Part model, mm, in its own coordinate system. A direction names the side the tool comes from. Round coordinates to 2 decimals unless told otherwise and drop trailing zeros. Order: outer loops, then holes, each group sorted by start corner. A loop starts at its lowest first (then second) coordinate and runs counter-clockwise, first axis right, second up. Notation, with made-up numbers: (-2.5, 41.25) - (41.5, 41.25) arc R18 ccw to (41.5, 67.25) - close; hole circle Ø8 at (26, 66). An arc over 180 degrees is marked (long way). Answer as a JSON object with one key per item and string values.
```python
from build123d import *

# Parameters (mm, degrees)
SKETCH1_R           = 200
SKETCH1_R_2         = 195
BOSS_EXTRUDE1_DEPTH = 137
SKETCH2_W           = 16
SKETCH2_H           = 10
CUT_EXTRUDE1_DEPTH  = 70.5


with BuildPart() as part:
    # Sketch1 → Boss-Extrude1 (new body)
    with BuildSketch(Plane(origin=(0, 0, 0), x_dir=(1, 0, 0), z_dir=(0, 1, 0))):
        with Locations(Location((0, 0, 0), (0, 0, 270))):
            Circle(SKETCH1_R)
        with Locations(Location((0, 0, 0), (0, 0, 270))):
            Circle(SKETCH1_R_2, mode=Mode.SUBTRACT)
    extrude(amount=BOSS_EXTRUDE1_DEPTH)

    # Sketch2 → Cut-Extrude1 (cut, symmetric)
    with BuildSketch(Plane(origin=(-200, 0, 0), x_dir=(0, 0, -1), z_dir=(1, 0, 0))):
        with Locations((52.378156189, 19.62104378)):
            Rectangle(SKETCH2_W, SKETCH2_H)
    extrude(amount=CUT_EXTRUDE1_DEPTH, both=True, mode=Mode.SUBTRACT)


solid = part.part
```
Item 1: Drop flat-ended pins along their axis: P1, Ø4, axis at x = -18, y = 45, coming from the -Z side; P2, Ø5, axis at x = 76, y = 83, coming from the +Z side; P3, Ø1.5, axis at x = -75, y = 45.5, coming from the -Z side. Give the stop position or say it passes through.
Taken from the geometry:
{"P1": "z = -199.36", "P2": "z = 186", "P3": "z = -185.71"}
Item 2: Cut at A-A (x = 0). Write the cut outline in (y, z).
Taken from the geometry:
{"outline": "(0, -200) - (137, -200) - (137, -195) - (0, -195) - close; (0, 195) - (137, 195) - (137, 200) - (0, 200) - close"}
Item 3: Two-plate mould, pull along X, no slides. Class faces 3 (the cylindrical face through (60.075, 67.541, 190.764)), 4 (the cylindrical face through (-173, 67.54, 89.98)), 5 (the flat face through (-190, 24.621, -52)): pulls with the +X half, pulls with the -X half, needs draft (parallel to the pull), parting line crosses it, or undercut.
Taken from the geometry:
{"face 3": "parting line crosses it", "face 4": "undercut", "face 5": "needs draft"}
Item 4: Cut at B-B (z = 0). Write the cut outline in (x, y), plus the area to 3 significant figures.
Taken from the geometry:
{"outline": "(-200, 0) - (-195, 0) - (-195, 137) - (-200, 137) - close; (195, 0) - (200, 0) - (200, 137) - (195, 137) - close", "area": "1,370 mm2"}
Item 5: Probe L1, parallel to Z at x = 3, y = 108; L2, parallel to X at y = 102.5, z = 0; L3, parallel to X at y = 125, z = -86. List the from-to ranges inside material, lowest first. Write a range as from..to.
Taken from the geometry:
{"L1": "-199.98..-194.98, 194.98..199.98", "L2": "-200..-195, 195..200", "L3": "-180.57..-175.01, 175.01..180.57"}
Item 6: Cut at C-C (y = 59). Write the cut outline in (x, z).
Taken from the geometry:
{"outline": "circle Ø400 at (0, 0); hole circle Ø390 at (0, 0)"}
Item 7: Tool access for faces 1 (the flat face through (-190, 14.621, -52)), 2 (the flat face through (-44, 137, 192)): list every direction of +Z, -Z, +X, -X, +Y, -Y with a clear straight run to the whole face (end or side of a thin tool).
Taken from the geometry:
{"face 1": "-X", "face 2": "+Z, -Z, +X, -X, +Y"}
